from build123d import *

# Parameters (mm, degrees)
SKETCH1_R               = 2.5
SKETCH1_R_2             = 14.26
BOSS_EXTRUDE1_DEPTH     = 3.3
SKETCH1_3_R             = 12.91
SALIENTE_EXTRUIR1_DEPTH = 3.3


with BuildPart() as part:
    # Sketch1 → Boss-Extrude1 (new body)
    with BuildSketch(Plane(origin=(0, 0, 0), x_dir=(1, 0, 0), z_dir=(0, 1, 0))):
        with BuildLine():
            Line((-117, 10), (-117, -60))
            ThreePointArc((-117, -60), (-97, -80), (-77, -60))
            Line((-77, -60), (-77, -10))
            Line((-77, -10), (77, -10))
            Line((77, -10), (77, -60))
            ThreePointArc((77, -60), (97, -80), (117, -60))
            Line((117, -60), (117, 10))
            Line((117, 10), (-117, 10))
        make_face()
        with BuildLine():
            ThreePointArc((77, -2.368543856), (73.7, 0), (77, 2.368543856))
            Line((77, 2.368543856), (77, -2.368543856))
        make_face(mode=Mode.SUBTRACT)
        with Locations((-101.6, 0)):
            Circle(SKETCH1_R, mode=Mode.SUBTRACT)
        with Locations((-76.2, 0)):
            Circle(SKETCH1_R, mode=Mode.SUBTRACT)
        with Locations((-50.8, 0)):
            Circle(SKETCH1_R, mode=Mode.SUBTRACT)
        with Locations((-25.4, 0)):
            Circle(SKETCH1_R, mode=Mode.SUBTRACT)
        Circle(SKETCH1_R, mode=Mode.SUBTRACT)
        with Locations((25.4, 0)):
            Circle(SKETCH1_R, mode=Mode.SUBTRACT)
        with Locations((50.8, 0)):
            Circle(SKETCH1_R, mode=Mode.SUBTRACT)
        with Locations((-97, -60)):
            Circle(SKETCH1_R_2, mode=Mode.SUBTRACT)
        with Locations((101.6, 0)):
            Circle(SKETCH1_R, mode=Mode.SUBTRACT)
        with Locations((97, -60)):
            Circle(SKETCH1_R_2, mode=Mode.SUBTRACT)
    extrude(amount=BOSS_EXTRUDE1_DEPTH)

    # Sketch1<3> → Saliente-Extruir1 (add)
    with BuildSketch(Plane(origin=(0, 0, 0), x_dir=(1, 0, 0), z_dir=(0, 1, 0))):
        with BuildLine():
            Line((-117, 30), (-117, 10))
            Line((-117, 10), (-77, 10))
            Line((-77, 10), (-77, 30))
            ThreePointArc((-77, 30), (-97, 50), (-117, 30))
        make_face()
        with Locations((-97, 30)):
            Circle(SKETCH1_3_R, mode=Mode.SUBTRACT)
    extrude(amount=SALIENTE_EXTRUIR1_DEPTH)


solid = part.part
Read the model definition and answer for the solid it produces. Units are mm, in the model's axes. Coordinates: 2 decimals unless noted, no trailing zeros. Loops run counter-clockwise (first coordinate to the right, second up) from the corner with the lowest first, then second, coordinate; pieces in that order, holes last. Notation, with made-up numbers: (71.25, 44) -> (86.25, 44) arc R35 cw to (86.25, 78) -> close; hole circle Ø8 at (-21.75, 83). An arc over 180 degrees is marked (long way). Answer in a Markdown table with one row per item.
Item 1: A cutting plane is placed at D-D on z = 54.5. Determine the outline of the cut face in (x, y).
Returned:
| item | result |
|---|---|
| outline | (-117, 0) -> (-110.16, 0) -> (-110.16, 3.3) -> (-117, 3.3) -> close; (-83.84, 0) -> (-77, 0) -> (-77, 3.3) -> (-83.84, 3.3) -> close; (77, 0) -> (83.84, 0) -> (83.84, 3.3) -> (77, 3.3) -> close; (110.16, 0) -> (117, 0) -> (117, 3.3) -> (110.16, 3.3) -> close |
Item 2: For a pull along X with two mould halves and no side action, classify faces 1 (the cylindrical face through (-97, 2, -50)), 2 (the flat face through (-9, 0, 5)), 3 (the cylindrical face through (27.71, 1.63, 0.96)) as released by +X, released by -X, zero draft, split by the parting line, or undercut.
Returned:
| item | result |
|---|---|
| face 1 | split by the parting line |
| face 2 | zero draft |
| face 3 | undercut |
Item 3: Each of these flat-tipped pins is pushed along its axis until it touches: P1, Ø4, axis at x = 25.4, z = 0, coming from the +Y side; P2, Ø1, axis at x = -35.5, y = 0.5, coming from the -Z side; P3, Ø1.6, axis at y = 1.5, z = -20.5, coming from the +X side. Where does it stop, or does it pass through?
Returned:
| item | result |
|---|---|
| P1 | passes through |
| P2 | stops at z = -10 |
| P3 | stops at x = -77 |
Item 4: Straight lines are drawn through the part: line 1 along Z through (x, y) = (-97, 1.6); line 2 along X through (y, z) = (0.75, 34.5); line 3 along Z through (x, y) = (-76.2, 2.6). For each, find the intervals that lie inside material, in ascending order. Write a range as [from, to].
Returned:
| item | result |
|---|---|
| line 1 | z = [-50, -42.91], [-17.09, 45.74], [74.26, 80] |
| line 2 | x = [-117, -77], [77, 117] |
| line 3 | z = [-10, -2.5], [2.5, 10] |
Item 5: A cutting plane is placed at C-C on z = 39.5. Determine the outline of the cut face in (x, y), plus the area to 3 significant figures.
Returned:
| item | result |
|---|---|
| outline | (-117, 0) -> (-77, 0) -> (-77, 3.3) -> (-117, 3.3) -> close; (77, 0) -> (117, 0) -> (117, 3.3) -> (77, 3.3) -> close |
| area | 264 mm^2 |
Item 6: A cutting plane is placed at A-A on x = 50.8. Determine the outline of the cut face in (y, z).
Returned:
| item | result |
|---|---|
| outline | (0, -10) -> (3.3, -10) -> (3.3, -2.5) -> (0, -2.5) -> close; (0, 2.5) -> (3.3, 2.5) -> (3.3, 10) -> (0, 10) -> close |
Item 7: A cutting plane is placed at B-B on y = 2.7. Give the number of separate pieces and of enclosed holes in the cut face, plus the area to 3 significant figures.
Returned:
| item | result |
|---|---|
| separate pieces | 1 |
| enclosed holes | 12 |
| area | 9,390 mm^2 |
